```python
from build123d import *

# Parameters (mm, degrees)
F0_R     = 10
F3_R     = 10
F4_DEPTH = 25
F5_R     = 2.5
F6_DEPTH = 25
F7_DEPTH = 25


with BuildPart() as f2:
    # F2: sweep along a path in F1
    with BuildLine(Plane.YZ) as f2_path:
        Line((45.0143888593, 63.3423924446), (13.3935455233, 58.710038662))
        ThreePointArc((13.3935455233, 58.710038662), (3.5423817202, 47.2169391208), (0, 32.5))
        Line((0, 32.5), (0, 0))
        Line((0, 0), (0, -32.5))
    # F0 (on Top) → F2 (sweep)
    with BuildSketch(Plane.XY):
        Circle(F0_R)
    sweep(path=f2_path.line, transition=Transition.RIGHT)

    # F3 (on face) → F4 (join)
    with BuildSketch(Plane(origin=(0, 0, -32.5), x_dir=(1, 0, 0), z_dir=(0, 0, -1))):
        Circle(F3_R)
    extrude(amount=F4_DEPTH)

    # F5 (on Right) → F6 (cut)
    with BuildSketch(Plane.YZ):
        with Locations((0, -45)):
            Circle(F5_R)
    extrude(amount=-F6_DEPTH, mode=Mode.SUBTRACT)

    # F7 (cut): a face of the model
    f7_faces = [f2.faces().sort_by_distance(p)[0] for p in [
        (0, 0, -45),
    ]]
    extrude(f7_faces, amount=-F7_DEPTH, mode=Mode.SUBTRACT)


solid = f2.part
```
Check sheet for the modelled part. Datum: model origin and axes. Units: mm. A direction names the side the tool comes from. Round coordinates to 2 decimals unless told otherwise and drop trailing zeros. Loops run counter-clockwise (first coordinate to the right, second up) from the corner with the lowest first, then second, coordinate; pieces in that order, holes last. Notation, with made-up numbers: (-37.5, 57) - (-25.5, 57) arc R22 ccw to (-25.5, 81) - close; hole circle Ø3 at (0.5, 64.5). An arc over 180 degrees is marked (long way). Write item = value, one per line. Start each with the question number.
Q1. Section check A-A (z = -17). Record the boundary of the cut face in (x, y).
Q2. Depth check by flat-ended pin: P1, Ø1.5, axis at x = 3, z = 35, coming from the -Y side; P2, Ø4, axis at y = 6, z = -8.5, coming from the +X side; P3, Ø12, axis at x = 2.5, z = 32.5, coming from the +Y side. Enter the tip coordinate at first touch or a pass-through.
Q3. Section check B-B (z = -45). Record the boundary of the cut face in (x, y), plus the area to 3 significant figures.
Q4. Thickness scan on L1, parallel to Y at x = -3, z = -45; L2, parallel to Y at x = -0.5, z = 9.5; L3, parallel to Y at x = -3.75, z = -44. Record the ranges inside material, lowest first.
Q5. Access from +Z, -Z, +X, -X, +Y, -Y to the whole of each face (thin tool, end or side, straight path). Record for faces 1 (the face through (0.14, 45.035, 63.204)), 2 (the face through (-2.17, 9.76, -11.87)).
Derived:
q1.outline = circle Ø20 at (0, 0)
q2.P1 = -9.67
q2.P2 = 9.17
q2.P3 = 10.72
q3.outline = (-9.68, -2.5) arc R10 ccw to (9.68, -2.5) - close; (-9.68, 2.5) - (9.68, 2.5) arc R10 ccw to start
q3.area = 215 mm^2
q4.L1 = -9.54 to -2.5, 2.5 to 9.54
q4.L2 = -9.99 to 9.99
q4.L3 = -9.27 to -2.29, 2.29 to 9.27
q5.face_1 = +Z, +X, -X, +Y
q5.face_2 = -Z
